The listing builds one solid part. Answer for the finished solid, in the listing's coordinates (mm). Face numbers are marked on the shaded views. A direction names the side the tool comes from. Give positions to 0.01 mm unless a question says otherwise; leave off trailing zeros. Loops run counter-clockwise (first coordinate to the right, second up) from the corner with the lowest first, then second, coordinate; pieces in that order, holes last. Notation, with made-up numbers: (-10.5, 56.5) - (4.5, 56.5) arc R18 cw to (4.5, 87.5) - close; hole circle Ø3 at (69.5, 77.25). An arc over 180 degrees is marked (long way). Write item = value, one per line. Start each with the question number.
1) Which of the six approach directions +Z, -Z, +X, -X, +Y, -Y give full straight-line access (tool end or side, diameter ignored) to the marked faces 1, 2 and 3?
2) The part is cut by section C-C on y = 201.5. Write down the section's boundary in (x, z), plus the area to 3 significant figures.
3) The mould has two halves that part along X. Classify the marked faces 4, 5, 6 and 7: +X half, -X half, draft (parallel to the pull), parting line (faces both ways), or undercut.
4) The part is cut by section B-B on z = 11. Write down the section's boundary in (x, y), plus the area to 3 significant figures.
5) The part is cut by section A-A on x = 151. Write down the section's boundary in (y, z).
6) The part is cut by section D-D on y = -122. Write down the section's boundary in (x, z), plus the area to 3 significant figures.
7) Consider probe 1 along Y at (x, z) = (193, 19); probe 2 along X at (y, z) = (28, 59); probe 3 along Y at (x, z) = (173, 37). Determine where each line is inside the solid, lowest interval first.
from build123d import *

# Parameters (mm, degrees)
F0_W     = 500
F0_H     = 500
F1_DEPTH = 80
F2_W     = 20
F2_H     = 30
F2_W_2   = 60
F2_H_2   = 50
F2_W_3   = 140
F3_DEPTH = 60
F4_W     = 160
F4_H     = 50
F5_DEPTH = 190
F6_W     = 60
F6_H     = 225
F7_DEPTH = 60


with BuildPart() as f1:
    # F0 (on Top) → F1 (new body)
    with BuildSketch(Plane.XY):
        Rectangle(F0_W, F0_H)
    extrude(amount=F1_DEPTH)

    # F2 (on face) → F3 (cut)
    with BuildSketch(Plane.XY.offset(80)):
        Polygon((-190, 105), (-210, 105), (-210, -105), (-190, -105), (-190, -75), (-190, -45), (-190, 45), (-190, 75), align=None)
        with Locations((-180, 60)):
            Rectangle(F2_W, F2_H)
        with Locations((-180, -60)):
            Rectangle(F2_W, F2_H)
        Polygon((-70, 75), (-140, 75), (-140, 45), (-130, 45), (-70, 45), align=None)
        Polygon((-140, -45), (-140, -75), (-70, -75), (-70, -45), (-130, -45), align=None)
        Polygon((140, 45), (140, 75), (70, 75), (70, 45), (130, 45), align=None)
        Polygon((70, -75), (140, -75), (140, -45), (130, -45), (70, -45), align=None)
        with Locations((180, 60)):
            Rectangle(F2_W, F2_H)
        Polygon((210, 105), (190, 105), (190, 75), (190, 45), (190, -45), (190, -75), (190, -105), (210, -105), align=None)
        with Locations((180, -60)):
            Rectangle(F2_W, F2_H)
        with Locations((-100, 0)):
            Rectangle(F2_W_2, F2_H_2)
        Rectangle(F2_W_3, F2_H_2)
        with Locations((100, 0)):
            Rectangle(F2_W_2, F2_H_2)
    extrude(amount=-F3_DEPTH, mode=Mode.SUBTRACT)

    # F4 (on face) → F5 (cut)
    with BuildSketch(Plane.XY.offset(80)):
        with Locations((-130, 195)):
            Rectangle(F4_W, F4_H)
        with Locations((130, 195)):
            Rectangle(F4_W, F4_H)
        with Locations((130, -195)):
            Rectangle(F4_W, F4_H)
        with Locations((-130, -195)):
            Rectangle(F4_W, F4_H)
    extrude(amount=-F5_DEPTH, mode=Mode.SUBTRACT)

    # F6 (on face) → F7 (cut)
    with BuildSketch(Plane.XY.offset(80)):
        with Locations((1.1277186871, -137.5)):
            Rectangle(F6_W, F6_H)
    extrude(amount=-F7_DEPTH, mode=Mode.SUBTRACT)


solid = f1.part
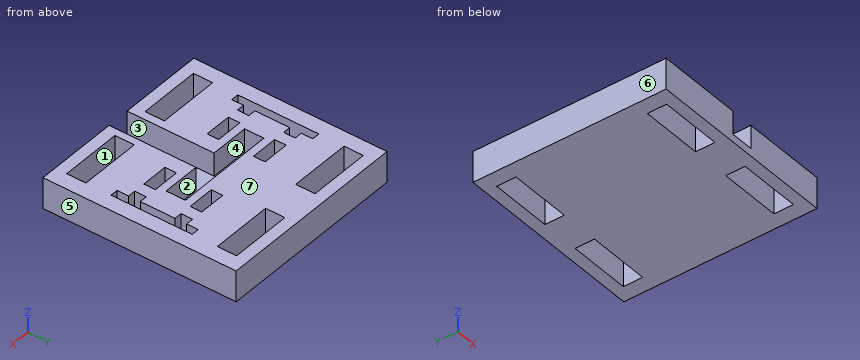
Answer below:
q1.face_1 = +Z, -Z
q1.face_2 = +Z
q1.face_3 = +Z, -Y
q2.outline = (-250, 0) - (-210, 0) - (-210, 80) - (-250, 80) - close; (-50, 0) - (50, 0) - (50, 80) - (-50, 80) - close; (210, 0) - (250, 0) - (250, 80) - (210, 80) - close
q2.area = 14,400 mm2
q3.face_4 = undercut
q3.face_5 = +X half
q3.face_6 = -X half
q3.face_7 = draft
q4.outline = (-250, -250) - (250, -250) - (250, 250) - (-250, 250) - close; hole (-210, -220) - (-50, -220) - (-50, -170) - (-210, -170) - close; hole (-210, 170) - (-50, 170) - (-50, 220) - (-210, 220) - close; hole (50, -220) - (210, -220) - (210, -170) - (50, -170) - close; hole (50, 170) - (210, 170) - (210, 220) - (50, 220) - close
q4.area = 218,000 mm2
q5.outline = (-250, 0) - (-220, 0) - (-220, 80) - (-250, 80) - close; (-170, 0) - (170, 0) - (170, 80) - (-170, 80) - close; (220, 0) - (250, 0) - (250, 80) - (220, 80) - close
q6.outline = (-250, 0) - (250, 0) - (250, 80) - (31.13, 80) - (31.13, 20) - (-28.87, 20) - (-28.87, 80) - (-250, 80) - close
q6.area = 36,400 mm2
q7.probe_1 = -250 to -220, -170 to 170, 220 to 250
q7.probe_2 = -250 to -210, -190 to 190, 210 to 250
q7.probe_3 = -250 to -220, -170 to -75, -45 to 45, 75 to 170, 220 to 250
